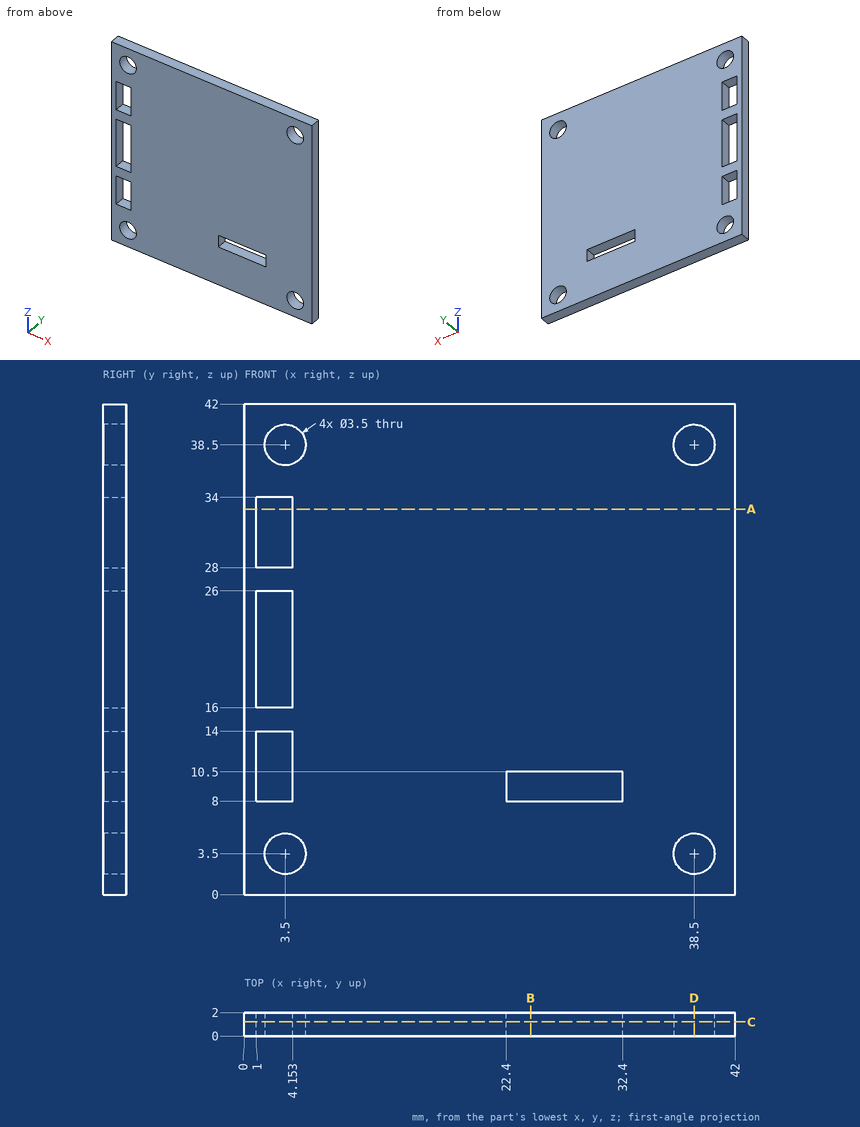
Design review of the part shown in the three views and the two pictorial views. Dimensions are in mm from the part's minimum x, y and z. Give positions to 0.01 mm unless a question says otherwise; leave off trailing zeros. Loops run counter-clockwise (first coordinate to the right, second up) from the corner with the lowest first, then second, coordinate; pieces in that order, holes last. Notation, with made-up numbers: (-37.5, 29) - (-2.5, 29) arc R27 cw to (-2.5, 58) - close; hole circle Ø6 at (73.5, 47). An arc over 180 degrees is marked (long way). Answer as a JSON object with one key per item and string values.
Q1. Add section A-A on z = 33. State the section outline as (x, y) points.
Worked out:
{"outline": "(0, 0) - (1, 0) - (1, 2) - (0, 2) - close; (4.15, 0) - (42, 0) - (42, 2) - (4.15, 2) - close"}
Q2. Add section D-D on x = 38.5. State the section outline as (y, z) points.
Worked out:
{"outline": "(0, 0) - (2, 0) - (2, 1.75) - (0, 1.75) - close; (0, 5.25) - (2, 5.25) - (2, 36.75) - (0, 36.75) - close; (0, 40.25) - (2, 40.25) - (2, 42) - (0, 42) - close"}
Q3. Add section B-B on x = 24.5. State the section outline as (y, z) points.
Worked out:
{"outline": "(0, 0) - (2, 0) - (2, 8) - (0, 8) - close; (0, 10.5) - (2, 10.5) - (2, 42) - (0, 42) - close"}
Q4. To check wall thickness, follow line 1 along X through (y, z) = (0.8, 38.5); line 2 along X through (y, z) = (0.9, 23). State the ranges of each line that lie inside material, in increasing order.
Worked out:
{"line 1": "x = 0 to 1.75, 5.25 to 36.75, 40.25 to 42", "line 2": "x = 0 to 1, 4.15 to 42"}
Q5. Insertion check: pin 1 (3 mm diameter, centred on x = 38.5, z = 3.5, fed in from +Y). The pin has a flat end and moves straight along its axis. Give the tip position at first contact, or say it passes through.
Worked out:
{"pin 1": "passes through"}
Q6. Add section C-C on y = 1.2. Count the separate pieces of the cut face and the enclosed holes in it, plus the area to 3 significant figures.
Worked out:
{"separate pieces": "1", "enclosed holes": "8", "area": "1,630 mm^2"}
